Geometry check sheet. Reference: the model listing, model coordinates, mm. A direction names the side the tool comes from. Coordinates: 2 decimals unless noted, no trailing zeros. Loops run counter-clockwise (first coordinate to the right, second up) from the corner with the lowest first, then second, coordinate; pieces in that order, holes last. Notation, with made-up numbers: M -6.75,-37 L 23.25,-37 A34 cw 23.25,-2 Z; hole C 63.5,25 d9. An arc over 180 degrees is marked long. One line per question, with ' | ' between items. Start each with the question number.
from build123d import *

# Parameters (mm, degrees)
F1_DEPTH  = 4
F3_DEPTH  = 55
F4_R      = 2.5
F5_DEPTH  = 2
F6_R      = 1.15
F7_DEPTH  = 2
F9_DEPTH  = 2.5
F10_R     = 1.7
F11_DEPTH = 1.5
F12_R     = 1.7
F13_DEPTH = 1.5
F15_DEPTH = 8
F17_DEPTH = 7
F18_R     = 2.6
F19_DEPTH = 6.5
F20_R     = 2.6
F21_DEPTH = 6.5
F22_W     = 110
F22_H     = 35
F23_DEPTH = 2.45


with BuildPart() as f1:
    # F0 (on Top) → F1 (new body)
    with BuildSketch(Plane.XY):
        with BuildLine():
            Line((-0.0348270737, 83.6430855933), (-60.0348270737, 83.6430855933))
            Line((-60.0348270737, 83.6430855933), (-60.0348270737, -26.3569144067))
            ThreePointArc((-60.0348270737, -26.3569144067), (-56.8036121084, -34.9342589227), (-48.7162364666, -39.2477197521))
            Line((-48.7162364666, -39.2477197521), (58.5887347718, -53.2440203484))
            Line((58.5887347718, -53.2440203484), (59.1074373156, -53.3116772019))
            ThreePointArc((59.1074373156, -53.3116772019), (62.8011202697, -51.776520456), (65.9774464875, -54.2077653548))
            Line((65.9774464875, -54.2077653548), (66.2837635334, -54.2477197521))
            Line((66.2837635334, -54.2477197521), (66.2837635334, -34.2477197521))
            Line((66.2837635334, -34.2477197521), (-0.0348270737, 83.6430855933))
        make_face()
        with BuildLine():
            Line((59.1074373156, -53.3116772019), (58.5887347718, -53.2440203484))
            Line((58.5887347718, -53.2440203484), (58.3714151196, -54.9101376817))
            ThreePointArc((58.3714151196, -54.9101376817), (58.6504322817, -54.0699295678), (59.1074373156, -53.3116772019))
        make_face()
        with BuildLine():
            Line((66.2835221478, -55.6989786465), (66.2837635334, -54.2477197521))
            Line((66.2837635334, -54.2477197521), (65.9774464875, -54.2077653548))
            ThreePointArc((65.9774464875, -54.2077653548), (66.2020782301, -54.9386771517), (66.2835221478, -55.6989786465))
        make_face()
        with BuildLine():
            Line((65.9774464875, -54.2077653548), (59.1074373156, -53.3116772019))
            ThreePointArc((59.1074373156, -53.3116772019), (58.6504322817, -54.0699295678), (58.3714151196, -54.9101376817))
            ThreePointArc((58.3714151196, -54.9101376817), (61.8425650137, -59.7185156245), (66.2835073084, -55.7881961))
            Line((66.2835073084, -55.7881961), (66.2835221478, -55.6989786465))
            ThreePointArc((66.2835221478, -55.6989786465), (66.2020782301, -54.9386771517), (65.9774464875, -54.2077653548))
        make_face()
        with BuildLine():
            ThreePointArc((66.2837635334, -55.7429221007), (66.2837031866, -55.7209500421), (66.2835221478, -55.6989786465))
            Line((66.2835221478, -55.6989786465), (66.2835073084, -55.7881961))
            ThreePointArc((66.2835073084, -55.7881961), (66.2836994767, -55.7655594629), (66.2837635334, -55.7429221007))
        make_face()
        with BuildLine():
            ThreePointArc((65.9774464875, -54.2077653548), (62.8011202697, -51.776520456), (59.1074373156, -53.3116772019))
            Line((59.1074373156, -53.3116772019), (65.9774464875, -54.2077653548))
        make_face()
    extrude(amount=F1_DEPTH)

    # F2 (on face) → F3 (join)
    with BuildSketch(Plane.XY.offset(4)):
        with BuildLine():
            ThreePointArc((-48.4575580984, -37.2645189297), (-55.300722103, -33.6146674587), (-58.0348270737, -26.3569144067))
            Line((-58.0348270737, -26.3569144067), (-58.0348270737, 83.6430855933))
            Line((-58.0348270737, 83.6430855933), (-60.0348270737, 83.6430855933))
            Line((-60.0348270737, 83.6430855933), (-60.0348270737, -26.3569144067))
            ThreePointArc((-60.0348270737, -26.3569144067), (-56.8036121084, -34.9342589227), (-48.7162364666, -39.2477197521))
            Line((-48.7162364666, -39.2477197521), (-48.4575580984, -37.2645189297))
        make_face()
        Polygon((-0.0348270737, 83.6430855933), (-2.3295637346, 83.6430855933), (59.1961841109, -25.7277544167), (66.2837635334, -34.2477197521), align=None)
    extrude(amount=F3_DEPTH)

    # F4 (on face) → F5 (cut, through all)
    with BuildSketch(Plane(origin=(-60.0348270737, 0, 0), x_dir=(0, -1, 0), z_dir=(-1, 0, 0))):
        with Locations((23.3569144067, 41.5)):
            Circle(F4_R)
        with Locations((-74.6430855933, 41.5)):
            Circle(F4_R)
    extrude(amount=-F5_DEPTH, mode=Mode.SUBTRACT)

    # F6 (on face) → F7 (cut)
    with BuildSketch(Plane.XY.offset(4)):
        with Locations((62.2837635334, -55.7429221007)):
            Circle(F6_R)
    extrude(amount=-F7_DEPTH, mode=Mode.SUBTRACT)

    # F8 (on face) → F9 (cut)
    with BuildSketch(Plane.XY.offset(4)):
        Polygon((-43.2614056757, -13.3569144067), (-46.7255072909, -13.3569144067), (-48.4575580984, -16.3569144067), (-46.7255072909, -19.3569144067), (-43.2614056757, -19.3569144067), (-41.5293548681, -16.3569144067), align=None)
        Polygon((16.7385943243, -13.3569144067), (13.2744927091, -13.3569144067), (11.5424419016, -16.3569144067), (13.2744927091, -19.3569144067), (16.7385943243, -19.3569144067), (18.4706451319, -16.3569144067), align=None)
    extrude(amount=-F9_DEPTH, mode=Mode.SUBTRACT)

    # F10 (on face) → F11 (cut, through all)
    with BuildSketch(Plane.XY.offset(1.5)):
        with Locations((15.0065435167, -16.3569144067)):
            Circle(F10_R)
    extrude(amount=-F11_DEPTH, mode=Mode.SUBTRACT)

    # F12 (on face) → F13 (cut, through all)
    with BuildSketch(Plane.XY.offset(1.5)):
        with Locations((-44.9934564833, -16.3569144067)):
            Circle(F12_R)
    extrude(amount=-F13_DEPTH, mode=Mode.SUBTRACT)

    # F14 (on face) → F15 (join)
    with BuildSketch(Plane.XY.offset(59)):
        with BuildLine():
            ThreePointArc((-52.7673478203, -9.3778442451), (-51.4986965275, -8.0981528472), (-51.0348270737, -6.3569144067))
            ThreePointArc((-51.0348270737, -6.3569144067), (-51.1491815724, -5.4695562268), (-51.4847725248, -4.6401828467))
            Line((-51.4847725248, -4.6401828467), (-51.6896180966, -4.3185852191))
            ThreePointArc((-51.6896180966, -4.3185852191), (-55.6052868974, -3.0246305403), (-58.0348270737, -6.3569143518))
            ThreePointArc((-58.0348270737, -6.3569143518), (-56.3204013937, -9.3671842197), (-52.856698827, -9.4283775088))
            Line((-52.856698827, -9.4283775088), (-52.7673478203, -9.3778442451))
        make_face()
        with BuildLine():
            Line((-51.6896180966, -4.3185852191), (-51.4847725248, -4.6401828467))
            ThreePointArc((-51.4847725248, -4.6401828467), (-51.5828126312, -4.4765924312), (-51.6896180966, -4.3185852191))
        make_face()
        with BuildLine():
            ThreePointArc((-58.0348270737, -6.3569143518), (-55.6052868974, -3.0246305403), (-51.6896180966, -4.3185852191))
            Line((-51.6896180966, -4.3185852191), (-58.0348270737, 5.6430855933))
            Line((-58.0348270737, 5.6430855933), (-58.0348270737, -6.3569143518))
        make_face()
        with BuildLine():
            Line((-58.0348270737, -12.3569144067), (-52.856698827, -9.4283775088))
            ThreePointArc((-52.856698827, -9.4283775088), (-56.3204013937, -9.3671842197), (-58.0348270737, -6.3569143518))
            Line((-58.0348270737, -6.3569143518), (-58.0348270737, -12.3569144067))
        make_face()
        with BuildLine():
            Line((-58.0348270737, 58.6430855933), (-58.0348270737, 53.6430855933))
            Line((-58.0348270737, 53.6430855933), (-53.4465181967, 55.3165883683))
            ThreePointArc((-53.4465181967, 55.3165883683), (-56.5892027611, 55.8094412023), (-58.0348270737, 58.6430855933))
        make_face()
        with BuildLine():
            Line((-53.2259221658, 55.3970467855), (-53.4465181967, 55.3165883683))
            ThreePointArc((-53.4465181967, 55.3165883683), (-53.3355452586, 55.3549671149), (-53.2259221658, 55.3970467855))
        make_face()
        with BuildLine():
            ThreePointArc((-58.0348270737, 58.6430855933), (-56.5892027611, 55.8094412023), (-53.4465181967, 55.3165883683))
            Line((-53.4465181967, 55.3165883683), (-53.2259221658, 55.3970467855))
            ThreePointArc((-53.2259221658, 55.3970467855), (-51.6338645457, 56.684918999), (-51.0348270737, 58.6430855933))
            ThreePointArc((-51.0348270737, 58.6430855933), (-51.1902368109, 59.6744516652), (-51.6426647732, 60.6142266912))
            ThreePointArc((-51.6426647732, 60.6142266912), (-55.5661931455, 61.9876758561), (-58.0348270737, 58.6430855933))
        make_face()
        with BuildLine():
            Line((-58.0348270737, 70.6430855933), (-58.0348270737, 58.6430855933))
            ThreePointArc((-58.0348270737, 58.6430855933), (-55.5661931455, 61.9876758561), (-51.6426647732, 60.6142266912))
            Line((-51.6426647732, 60.6142266912), (-58.0348270737, 70.6430855933))
        make_face()
    extrude(amount=-F15_DEPTH)

    # F16 (on face) → F17 (join)
    with BuildSketch(Plane.XY.offset(59)):
        with BuildLine():
            ThreePointArc((5.1432437589, 70.3590986219), (1.3150969821, 72.0555922251), (-1.3999848728, 68.86793967))
            ThreePointArc((-1.3999848728, 68.86793967), (-0.7360869019, 66.5821430027), (1.236164718, 65.2495326066))
            Line((1.236164718, 65.2495326066), (1.518343575, 65.1905478063))
            ThreePointArc((1.518343575, 65.1905478063), (4.3554664208, 65.9728286191), (5.5927848941, 68.6430855933))
            ThreePointArc((5.5927848941, 68.6430855933), (5.4785348868, 69.5300449986), (5.1432437589, 70.3590986219))
        make_face()
        with BuildLine():
            Line((-0.6419361775, 80.6430855933), (-1.3999848728, 68.86793967))
            ThreePointArc((-1.3999848728, 68.86793967), (1.3150969821, 72.0555922251), (5.1432437589, 70.3590986219))
            Line((5.1432437589, 70.3590986219), (-0.6419361775, 80.6430855933))
        make_face()
        with BuildLine():
            Line((8.9212866456, 63.6430855933), (5.1432437589, 70.3590986219))
            ThreePointArc((5.1432437589, 70.3590986219), (5.4785348868, 69.5300449986), (5.5927848941, 68.6430855933))
            ThreePointArc((5.5927848941, 68.6430855933), (4.3554664208, 65.9728286191), (1.518343575, 65.1905478063))
            Line((1.518343575, 65.1905478063), (8.9212866456, 63.6430855933))
        make_face()
        with BuildLine():
            Line((52.9593578497, -14.6409013336), (47.1741779383, -4.3569144067))
            Line((47.1741779383, -4.3569144067), (46.4675691299, -15.7187540374))
            ThreePointArc((46.4675691299, -15.7187540374), (49.3356306127, -12.9041816709), (52.9593578497, -14.6409013336))
        make_face()
        with BuildLine():
            ThreePointArc((52.9593578497, -14.6409013336), (49.3356306127, -12.9041816709), (46.4675691299, -15.7187540374))
            ThreePointArc((46.4675691299, -15.7187540374), (47.0023195828, -18.3067338942), (49.1940807829, -19.7831419097))
            ThreePointArc((49.1940807829, -19.7831419097), (52.1166281832, -19.0727811002), (53.4088990099, -16.3569144067))
            ThreePointArc((53.4088990099, -16.3569144067), (53.2946489962, -15.4699549767), (52.9593578497, -14.6409013336))
        make_face()
        with BuildLine():
            Line((56.7374007615, -21.3569144067), (52.9593578497, -14.6409013336))
            ThreePointArc((52.9593578497, -14.6409013336), (53.2946489962, -15.4699549767), (53.4088990099, -16.3569144067))
            ThreePointArc((53.4088990099, -16.3569144067), (52.1166281832, -19.0727811002), (49.1940807829, -19.7831419097))
            Line((49.1940807829, -19.7831419097), (56.7374007615, -21.3569144067))
        make_face()
    extrude(amount=-F17_DEPTH)

    # F18 (on face) → F19 (cut)
    with BuildSketch(Plane.XY.offset(59)):
        with Locations((-54.5348270737, -6.3569144067)):
            Circle(F18_R)
        with Locations((-54.5348270737, 58.6430855933)):
            Circle(F18_R)
    extrude(amount=-F19_DEPTH, mode=Mode.SUBTRACT)

    # F20 (on face) → F21 (cut)
    with BuildSketch(Plane.XY.offset(59)):
        with Locations((49.9088990099, -16.3569144067)):
            Circle(F20_R)
        with Locations((2.0927848941, 68.6430855933)):
            Circle(F20_R)
    extrude(amount=-F21_DEPTH, mode=Mode.SUBTRACT)

    # F22 (on face) → F23 (join)
    with BuildSketch(Plane(origin=(-60.0348270737, 0, 0), x_dir=(0, -1, 0), z_dir=(-1, 0, 0))):
        with Locations((-28.6430855933, 17.5)):
            Rectangle(F22_W, F22_H)
    extrude(amount=F23_DEPTH)


solid = f1.part
1. Sectioned sample at D-D (z = 54.5). State how many separate pieces and enclosed holes the cut face has, and give its area (3 significant figures).
2. Tool access check on faces 5 (the flat face through (3, 70, 52)), 6 (the flat face through (-54.794, 65.558, 55.056)), 7 (the cylindrical face through (47.31, -16.24, 55.8)). Record the directions out of +Z, -Z, +X, -X, +Y, -Y that give a thin tool (end or side, any length) a straight path to the whole face; none if there is none.
3. Sectioned sample at A-A (z = 24). Record the cut outline in (x, y), and give its area (3 significant figures).
4. Sectioned sample at B-B (z = 41.5). Record the cut outline in (x, y), and give its area (3 significant figures).
5. Depth check by flat-ended pin: pin 1 Ø3 at (x, z) = (15.5, 2.5) entering from -Y; pin 2 Ø1 at (y, z) = (-27.5, 51) entering from -X; pin 3 Ø4 at (y, z) = (-23.36, 41.5) entering from +X. Enter the tip coordinate at first touch or a pass-through.
6. Draft check along Z on faces 1 (the flat face through (-55, 60, 51)), 2 (the cylindrical face through (-0.756, 66.61, 55.549)), 3 (the flat face through (-12, 13, 0)), 4 (the flat face through (28.003, 29.723, 31.115)). Enter one of: +Z half, -Z half, draft (parallel to the pull), parting line (faces both ways), or undercut.
7. Sectioned sample at C-C (y = 31). Record the cut outline in (x, z).
8. Thickness scan on line 1 (Z direction, x = -45, y = 61.5); line 2 (X direction, y = 13.5, z = 52.5); line 3 (X direction, y = 40, z = 27.5). Record the ranges inside material, lowest first.
Result:
1) separate pieces: 2 | enclosed holes: 4 | area: 728 mm2
2) face 5: -Y | face 6: +Z, +Y | face 7: +Z
3) outline: M -62.48,-26.36 L -60.03,-26.36 A13 ccw -48.72,-39.25 L -48.46,-37.26 A11 cw -58.03,-26.36 L -58.03,83.64 L -62.48,83.64 Z; M -2.33,83.64 L 59.2,-25.73 L 66.28,-34.25 L -0.03,83.64 Z | area: 785 mm2
4) outline: M -60.03,-26.36 A13 ccw -48.72,-39.25 L -48.46,-37.26 A11 cw -58.03,-26.36 L -58.03,-25.86 L -60.03,-25.86 Z; M -60.03,-20.86 L -58.03,-20.86 L -58.03,72.14 L -60.03,72.14 Z; M -60.03,77.14 L -58.03,77.14 L -58.03,83.64 L -60.03,83.64 Z; M -2.33,83.64 L 59.2,-25.73 L 66.28,-34.25 L -0.03,83.64 Z | area: 495 mm2
5) pin 1: stops at y = -47.82 | pin 2: stops at x = -60.02 | pin 3: stops at x = 61.28
6) face 1: undercut | face 2: draft | face 3: -Z half | face 4: undercut
7) outline: M -62.48,0 L 29.58,0 L 29.58,59 L 27.28,59 L 27.28,4 L -58.03,4 L -58.03,59 L -60.03,59 L -60.03,35 L -62.48,35 Z
8) line 1: z = 0 to 4 | line 2: x = -60.03 to -58.03, 37.13 to 39.42 | line 3: x = -62.48 to -58.03, 22.22 to 24.52
